Check sheet for the drawn part. Datum: minimum x, y, z corner. Units: mm. Coordinates: 2 decimals unless noted, no trailing zeros. Return JSON: item names as keys, results as strings. Group by question number.
Q1. Section check A-A, the plane z = 1.5. Count the separate pieces of the cut face and the enclosed holes in it, then the cut area to 3 significant figures.
Q2. Go/stop test with flat-tipped pins: pin 1 Ø2.5 at (x, y) = (22, 10) entering from +Z; pin 2 Ø2.5 at (x, y) = (33.5, 2) entering from +Z; pin 3 Ø4.5 at (x, y) = (27, 15) entering from -Z. Record where each tip stops, or that it passes through.
Q3. Thickness scan on probe 1 along Y at (x, z) = (9, 0.7); probe 2 along Y at (x, z) = (9, 1.3); probe 3 along Z at (x, y) = (27, 5.25). Record the ranges inside material, lowest first.
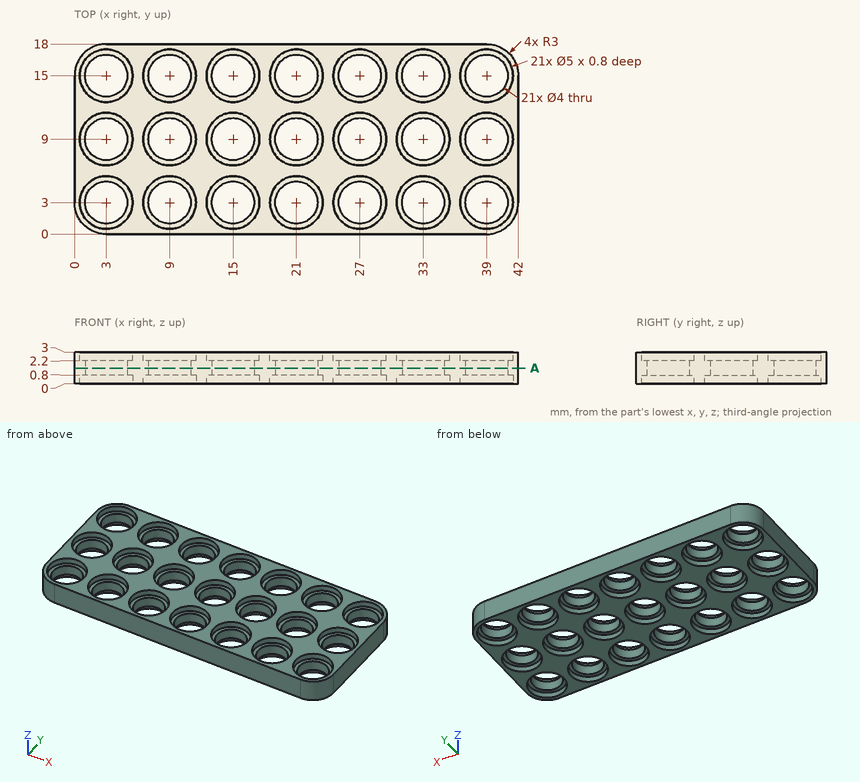
Numbers:
{
 "1": {"separate pieces": "1", "enclosed holes": "21", "area": "484 mm2"},
 "2": {"pin 1": "stops at z = 3", "pin 2": "stops at z = 2.2", "pin 3": "stops at z = 0.8"},
 "3": {"probe 1": "y = 0 to 0.5, 5.5 to 6.5, 11.5 to 12.5, 17.5 to 18", "probe 2": "y = 0 to 1, 5 to 7, 11 to 13, 17 to 18", "probe 3": "z = 0.8 to 2.2"}
}
